Model file for the job. Use its own axes, mm. Face numbers are marked on the shaded views. Give positions to 0.01 mm unless a question says otherwise; leave off trailing zeros. Write each loop counter-clockwise with the first axis right and the second up, starting at its lowest first coordinate (ties: lowest second). Pieces come first, ordered by that corner, then holes.
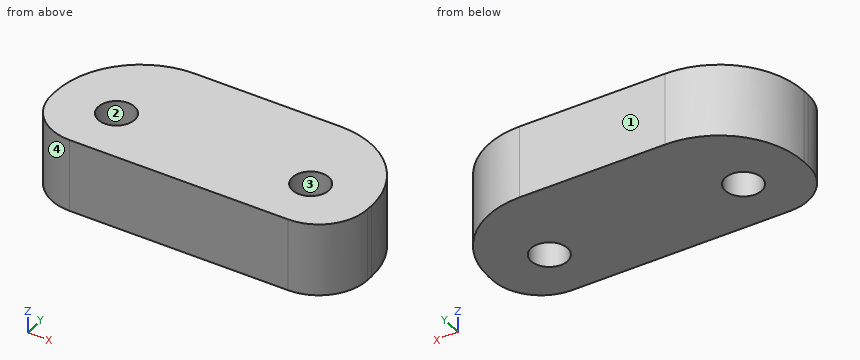
```python
from build123d import *

# Parameters (mm, degrees)
ESBO_O1_W                = 26
ESBO_O1_H                = 11.5
ESBO_O1_R                = 1.5
RESSALTO_EXTRUS_O1_DEPTH = 6
FILETE1_R                = 7
FILETE2_R                = 4


with BuildPart() as part:
    # Esboço1 → Ressalto-extrusão1 (new body)
    with BuildSketch(Plane.XY):
        Rectangle(ESBO_O1_W, ESBO_O1_H)
        with Locations((-8, -1.25)):
            Circle(ESBO_O1_R, mode=Mode.SUBTRACT)
        with Locations((8, -1.25)):
            Circle(ESBO_O1_R, mode=Mode.SUBTRACT)
    extrude(amount=RESSALTO_EXTRUS_O1_DEPTH)

    # Filete1
    filete1_edges = [part.edges().sort_by_distance(p)[0] for p in [
        (-13, 5.75, 3),
        (13, 5.75, 3),
    ]]
    fillet(filete1_edges, radius=FILETE1_R)

    # Filete2
    filete2_edges = [part.edges().sort_by_distance(p)[0] for p in [
        (-13, -5.75, 3),
        (13, -5.75, 3),
    ]]
    fillet(filete2_edges, radius=FILETE2_R)


solid = part.part
```
1. Slice it at A-A, the plane x = -6.75. Write the cut outline in (y, z), and give its area (3 significant figures).
Calculated:
outline: (-5.75, 0) - (-2.08, 0) - (-2.08, 6) - (-5.75, 6) - close; (-0.42, 0) - (5.71, 0) - (5.71, 6) - (-0.42, 6) - close
area: 58.8 mm2
2. Slice it at D-D, the plane x = 8. Write the cut outline in (y, z).
Calculated:
outline: (-5.75, 0) - (-2.75, 0) - (-2.75, 6) - (-5.75, 6) - close; (0.25, 0) - (5.46, 0) - (5.46, 6) - (0.25, 6) - close
3. Slice it at C-C, the plane y = -1. Write the cut outline in (x, z).
Calculated:
outline: (-13, 0) - (-9.48, 0) - (-9.48, 6) - (-13, 6) - close; (-6.52, 0) - (6.52, 0) - (6.52, 6) - (-6.52, 6) - close; (9.48, 0) - (13, 0) - (13, 6) - (9.48, 6) - close
4. Probe probe 1 along X at (y, z) = (-1, 3.45); probe 2 along X at (y, z) = (0, 5.05); probe 3 along Y at (x, z) = (-8, 1.5). List the from-to ranges inside material, lowest first.
Calculated:
probe 1: x = -13 to -9.48, -6.52 to 6.52, 9.48 to 13
probe 2: x = -12.89 to -8.83, -7.17 to 7.17, 8.83 to 12.89
probe 3: y = -5.75 to -2.75, 0.25 to 5.46
5. Pull direction X, two halves, no side cores. Call the marked faces 1, 2, 3 and 4: +X half, -X half, draft (parallel to the pull), parting line (faces both ways), or undercut.
Calculated:
face 1: draft
face 2: undercut
face 3: undercut
face 4: -X half
6. Slice it at B-B, the plane z = 4.6. Write the cut outline in (x, y), and give its area (3 significant figures).
Calculated:
outline: (-13, -1.75) arc R4 ccw to (-9, -5.75) - (9, -5.75) arc R4 ccw to (13, -1.75) - (13, -1.25) arc R7 ccw to (6, 5.75) - (-6, 5.75) arc R7 ccw to (-13, -1.25) - close; hole circle Ø3 at (-8, -1.25); hole circle Ø3 at (8, -1.25)
area: 257 mm2
7. Pin check, flat tip, straight feed: P1, Ø3, axis at y = 0.5, z = 4, coming from the -X side. Stop position of the tip, or through.
Calculated:
P1: stops at x = -13
